CAD build for the part. Positions are in the model's coordinates, mm. A direction names the side the tool comes from. Give positions to 0.01 mm unless a question says otherwise; leave off trailing zeros. Loops run counter-clockwise (first coordinate to the right, second up) from the corner with the lowest first, then second, coordinate; pieces in that order, holes last.
```python
from build123d import *

# Parameters (mm, degrees)
BOSS_EXTRUDE1_DEPTH                               = 3.175
CSK_FOR_6_FLAT_HEAD_MACHINE_SCREW_100_D           = 4.3053
CSK_FOR_6_FLAT_HEAD_MACHINE_SCREW_100_DEPTH       = 3.175
CSK_FOR_6_FLAT_HEAD_MACHINE_SCREW_100_CSINK_D     = 7.0866
CSK_FOR_6_FLAT_HEAD_MACHINE_SCREW_100_CSINK_ANGLE = 100


with BuildPart() as part:
    # Sketch1 → Boss-Extrude1 (new body)
    with BuildSketch(Plane.XY):
        with BuildLine():
            Line((-129.2225, -27.397612764), (-129.2225, -75.892938058))
            Line((-129.2225, -75.892938058), (-63.036003441, -81.587899176))
            Line((-63.036003441, -81.587899176), (-51.562, -77.411703455))
            Line((-51.562, -77.411703455), (-51.562, -23.241))
            Line((-51.562, -23.241), (-123.825, -23.241))
            ThreePointArc((-123.825, -23.241), (-124.792433255, -23.184983239), (-125.746935831, -23.017681674))
            ThreePointArc((-125.746935831, -23.017681674), (-127.22324483, -25.415131417), (-129.2225, -27.397612764))
        make_face()
    extrude(amount=BOSS_EXTRUDE1_DEPTH)

    # CSK for #6 Flat Head Machine Screw (100)1
    with Locations(Plane.XY.offset(3.175)):
        with Locations((-123.300524074, -70.458632008), (-122.245302558, -29.869734201), (-57.342596045, -29.021596045), (-64.02512283, -74.422207293)):
            CounterSinkHole(CSK_FOR_6_FLAT_HEAD_MACHINE_SCREW_100_D / 2, CSK_FOR_6_FLAT_HEAD_MACHINE_SCREW_100_CSINK_D / 2, depth=CSK_FOR_6_FLAT_HEAD_MACHINE_SCREW_100_DEPTH, counter_sink_angle=CSK_FOR_6_FLAT_HEAD_MACHINE_SCREW_100_CSINK_ANGLE)


solid = part.part
```
1. Tool access for faces 1 (the face through (-96.6, -78.7, 1.6)), 2 (the face through (-87, -23.241, 2)): list every direction of +Z, -Z, +X, -X, +Y, -Y with a clear straight run to the whole face (end or side of a thin tool).
Responses:
face 1: +Z, -Z, -X, -Y
face 2: +Z, -Z, +X, +Y
2. Saw through at B-B, the plane x = -78. List the corners of the cut face in (y, z) (3 decimals), and give its area (3 significant figures).
Responses:
outline: (-80.3, 0) - (-23.241, 0) - (-23.241, 3.175) - (-80.3, 3.175) - close
area: 181 mm2
3. Saw through at C-C, the plane x = -102.5. List the corners of the cut face in (y, z) (3 decimals).
Responses:
outline: (-78.192, 0) - (-23.241, 0) - (-23.241, 3.175) - (-78.192, 3.175) - close
4. Probe line 1 along X through (y, z) = (-30.5, 0.2); line 2 along Y through (x, z) = (-122, 1.55); line 3 along X through (y, z) = (-74, 0.2). List the from-to ranges inside material, lowest first.
Responses:
line 1: x = -129.22 to -124.3, -120.19 to -58.91, -55.78 to -51.56
line 2: y = -76.51 to -72.17, -68.74 to -32.01, -27.73 to -23.24
line 3: x = -129.22 to -66.14, -61.91 to -51.56
5. Drop a flat-ended pin along its axis: pin 1 (5.5 mm diameter, centred on x = -123.3, y = -70.46, fed in from +Z). Give the stop position or say it passes through.
Responses:
pin 1: stops at z = 2.51
6. Pull direction Y, two halves, no side cores. Call faces 3 (the face through (-59.396, -28.375, 0.99)), 4 (the face through (-51.562, -51, 2)), 5 (the face through (-57.38, -79.53, 1.57)), 6 (the face through (-120.095, -29.775, 0.99)): released by +Y, released by -Y, zero draft, split by the parting line, or undercut.
Responses:
face 3: undercut
face 4: zero draft
face 5: released by -Y
face 6: undercut
7. Saw through at A-A, the plane z = 2.65. List the corners of the cut face in (x, y) (1 decimal), and give its area (3 significant figures).
Responses:
outline: (-129.2, -75.9) - (-63, -81.6) - (-51.6, -77.4) - (-51.6, -23.2) - (-123.8, -23.2) arc R8.4 cw to (-125.7, -23) arc R11.9 cw to (-129.2, -27.4) - close; hole circle Ø5.8 at (-123.3, -70.5); hole circle Ø5.8 at (-122.2, -29.9); hole circle Ø5.8 at (-64, -74.4); hole circle Ø5.8 at (-57.3, -29)
area: 4,200 mm2
